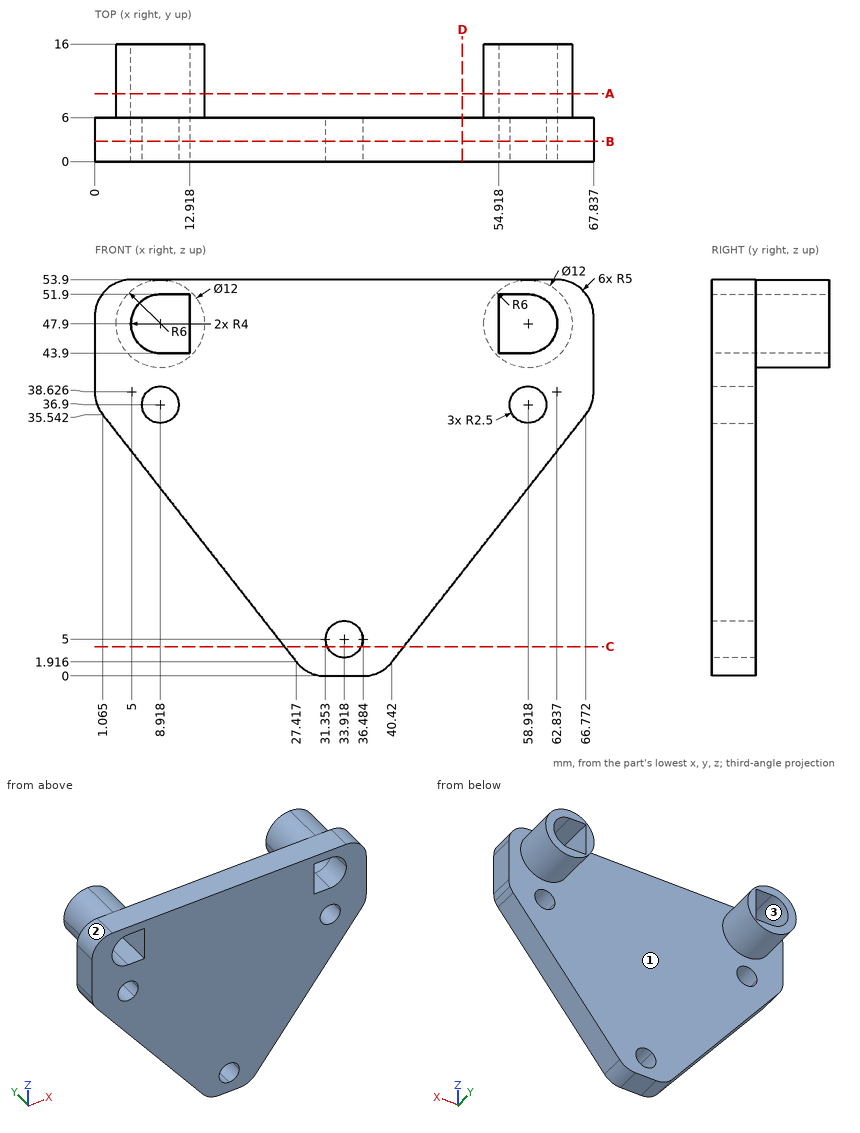
Design review of the part shown in the three views and the two pictorial views. Dimensions are in mm from the part's minimum x, y and z. Give positions to 0.01 mm unless a question says otherwise; leave off trailing zeros. Write each loop counter-clockwise with the first axis right and the second up, starting at its lowest first coordinate (ties: lowest second). Pieces come first, ordered by that corner, then holes. Notation, with made-up numbers: (18.5, 47) -> (38.5, 47) arc R16 ccw to (38.5, 63) -> close; hole circle Ø10 at (-36.75, 8). An arc over 180 degrees is marked (long way). Answer in a Markdown table with one row per item.
1) Add section C-C on z = 4. State the section outline as (x, y) points.
Worked answers:
| item | result |
|---|---|
| outline | (25.78, 0) -> (31.63, 0) -> (31.63, 6) -> (25.78, 6) -> close; (36.21, 0) -> (42.05, 0) -> (42.05, 6) -> (36.21, 6) -> close |
2) Mouldability with a two-part tool opening along Z and no side actions: class the marked faces 1, 2 and 3 as +Z half, -Z half, draft (parallel to the pull), parting line (faces both ways), or undercut.
Worked answers:
| item | result |
|---|---|
| face 1 | draft |
| face 2 | +Z half |
| face 3 | undercut |
3) Add section D-D on x = 50. State the section outline as (y, z) points.
Worked answers:
| item | result |
|---|---|
| outline | (0, 14.14) -> (6, 14.14) -> (6, 53.9) -> (0, 53.9) -> close |
4) For L1, parallel to X at y = 3.5, z = 37 (1 decimal); L2, parallel to X at y = 8.25, z = 45.5; L3, parallel to Y at x = 35, z = 35, list the stretches that pass through material, from the lowest coordinate up. Write a range as [from, to].
Worked answers:
| item | result |
|---|---|
| L1 | [0.3, 6.4], [11.4, 56.4], [61.4, 67.6] |
| L2 | [3.42, 5.72], [12.92, 14.42], [53.42, 54.92], [62.12, 64.42] |
| L3 | [0, 6] |
5) Add section A-A on y = 9.25. State the section outline as (x, z) points.
Worked answers:
| item | result |
|---|---|
| outline | circle Ø12 at (8.92, 47.9); circle Ø12 at (58.92, 47.9); hole (8.92, 43.9) -> (12.92, 43.9) -> (12.92, 51.9) -> (8.92, 51.9) arc R4 ccw to start; hole (54.92, 43.9) -> (58.92, 43.9) arc R4 ccw to (58.92, 51.9) -> (54.92, 51.9) -> close |
6) Clearance check with flat-ended pins moving along their axes: P1, Ø3, axis at y = 6.5, z = 18, coming from the +X side (1 decimal); P2, Ø9, axis at y = 5.5, z = 48.5, coming from the -X side; P3, Ø6, axis at y = 2.5, z = 25.5, coming from the +X side (1 decimal); P4, Ø1.5, axis at x = 55.5, y = 3, coming from the -Z side. State where each tip first meets the part, or that it passes through.
Worked answers:
| item | result |
|---|---|
| P1 | x = 54.1 |
| P2 | x = 0 |
| P3 | x = 61.3 |
| P4 | z = 20.2 |
7) Add section B-B on y = 2.75. State the section outline as (x, z) points (1 decimal).
Worked answers:
| item | result |
|---|---|
| outline | (0, 38.6) arc R5 ccw to (1.1, 35.5) -> (27.4, 1.9) arc R5 ccw to (31.4, 0) -> (36.5, 0) arc R5 ccw to (40.4, 1.9) -> (66.8, 35.5) arc R5 ccw to (67.8, 38.6) -> (67.8, 48.9) arc R5 ccw to (62.8, 53.9) -> (5, 53.9) arc R5 ccw to (0, 48.9) -> close; hole circle Ø5 at (8.9, 36.9); hole (8.9, 43.9) -> (12.9, 43.9) -> (12.9, 51.9) -> (8.9, 51.9) arc R4 ccw to start; hole circle Ø5 at (33.9, 5); hole (54.9, 43.9) -> (58.9, 43.9) arc R4 ccw to (58.9, 51.9) -> (54.9, 51.9) -> close; hole circle Ø5 at (58.9, 36.9) |
